```python
from build123d import *

# Parameters (mm, degrees)
ESTRUSIONE_ESTRUSIONE1_DEPTH = 140
SCHIZZO2_W                   = 160
SCHIZZO2_H                   = 100
TAGLIO_ESTRUSIONE1_DEPTH     = 140


with BuildPart() as part:
    # Schizzo1 → Estrusione-Estrusione1 (new body)
    with BuildSketch(Plane.XY):
        with BuildLine():
            Line((40, 40), (-40, 40))
            ThreePointArc((-40, 40), (-80, 0), (-40, -40))
            Line((-40, -40), (40, -40))
            Line((40, -40), (40, 40))
        make_face()
    extrude(amount=ESTRUSIONE_ESTRUSIONE1_DEPTH)

    # Schizzo2 → Taglio-Estrusione1 (cut)
    with BuildSketch(Plane(origin=(0, 40, 0), x_dir=(1, 0, 0), z_dir=(0, 1, 0))):
        with Locations((-80, -70)):
            Rectangle(SCHIZZO2_W, SCHIZZO2_H)
    extrude(amount=-TAGLIO_ESTRUSIONE1_DEPTH, mode=Mode.SUBTRACT)


solid = part.part
```
For this review, take the finished solid that the model builds, in its own axes (mm). A direction names the side the tool comes from. Coordinates: 2 decimals unless noted, no trailing zeros. Loops run counter-clockwise (first coordinate to the right, second up) from the corner with the lowest first, then second, coordinate; pieces in that order, holes last.
1. Add section B-B, the plane y = -24. Give the boundary of the cut face in (x, z).
2. Add section C-C, the plane z = 40.5. Give the boundary of the cut face in (x, y).
3. For line 1 (Z direction, x = -69, y = -8); line 2 (X direction, y = 33, z = 80); line 3 (X direction, y = 24.5, z = 6), list the stretches that pass through material, from the lowest coordinate up.
4. Insertion check: P1, Ø8, axis at y = 9.5, z = 76, coming from the -X side. The pin has a flat end and moves straight along its axis. Give the tip position at first contact, or say it passes through.
5. Add section A-A, the plane x = -18. Give the boundary of the cut face in (y, z), then the cut area to 3 significant figures.
6. Add section D-D, the plane x = -43. Give the boundary of the cut face in (y, z), then the cut area to 3 significant figures.
7. For faces 1 (the flat face through (40, -1, 69)), 2 (the flat face through (0, 1, 71)), list the 3-axis set-ups (+Z, -Z, +X, -X, +Y, -Y) from which the entire face can be reached by the end or side of a thin tool; tool diameter is ignored.
Result:
1. outline: (-72, 0) - (40, 0) - (40, 140) - (-72, 140) - (-72, 120) - (0, 120) - (0, 20) - (-72, 20) - close
2. outline: (0, -40) - (40, -40) - (40, 40) - (0, 40) - close
3. line 1: z = 0 to 20, 120 to 140
3. line 2: x = 0 to 40
3. line 3: x = -71.62 to 40
4. P1: stops at x = 0
5. outline: (-40, 0) - (40, 0) - (40, 20) - (-40, 20) - close; (-40, 120) - (40, 120) - (40, 140) - (-40, 140) - close
5. area: 3,200 mm2
6. outline: (-39.89, 0) - (39.89, 0) - (39.89, 20) - (-39.89, 20) - close; (-39.89, 120) - (39.89, 120) - (39.89, 140) - (-39.89, 140) - close
6. area: 3,190 mm2
7. face 1: +Z, -Z, +X, +Y, -Y
7. face 2: -X, +Y, -Y
